CAD build for the part. Positions are in the model's coordinates, mm. Give positions to 0.01 mm unless a question says otherwise; leave off trailing zeros. Order: outer loops, then holes, each group sorted by start corner. A loop starts at its lowest first (then second) coordinate and runs counter-clockwise, first axis right, second up.
Item 1: Wall check: L1, parallel to Y at x = 14.5, z = 0.75; L2, parallel to Y at x = 23.5, z = 2.25; L3, parallel to X at y = 1.5, z = 6.5. Give the ranges that are in metal, low to high.
Item 2: Band-saw the part on A-A on z = 5.5. Give the cut face in (x, y) (3 decimals).
Item 3: Band-saw the part on D-D on x = 14. Give the cut face in (y, z) (3 decimals).
Item 4: Band-saw the part on B-B on x = 27. Give the cut face in (y, z), plus the area to 3 significant figures.
Item 5: Two-plate mould, pull along Y, no slides. Class faces 1 (the flat face through (14, 10, 4)), 2 (the flat face through (19.82, 12.146, 3.55)), 3 (the flat face through (26.8, 1.5, 3.5)), 4 (the flat face through (29.2, 6, 4)): released by +Y, released by -Y, zero draft, split by the parting line, or undercut.
Item 6: Band-saw the part on C-C on y = 2.3. Give the cut face in (x, z) (3 decimals), plus the area to 3 significant figures.
Item 7: Flat gauge pins, fed straight in: P1, Ø1, axis at x = 16.5, z = 2.5, coming from the +Y side; P2, Ø1.5, axis at x = 9.5, z = 1, coming from the +Y side; P3, Ø3.5, axis at x = 15.5, z = 4.5, coming from the +Y side. Where does each tip first touch, or does it go through?
Autodesk Inventor part; units mm, degrees
ref_plane "YZ Plane" through (0, 0, 0) normal (1, 0, 0) x (0, 1, 0)
ref_plane "XZ Plane" through (0, 0, 0) normal (0, 1, 0) x (-1, 0, 0)
ref_plane "XY Plane" through (0, 0, 0) normal (0, 0, 1) x (1, 0, 0)
sketch "スケッチ1" plane through (0, 0, 0) normal (0, 0, 1) x (1, 0, 0)
  line L0 (0, 0) -> (24.2856, 0)
  line L1 (29.2, 2.9323) -> (29.2, 10)
  line L2 (28.3778, 10) -> (0, 10)
  line L3 (0, 10) -> (0, 0)
  circle A0 centre (23.5, 2.3) radius 1.25
  circle A1 centre (14, 2.3) radius 1.175
  line L4 (29.2, 2.9323) -> (24.2856, 0)
  line L5 (29.2, 10) -> (11.5467, 14.4273)
  line L6 (11.5467, 14.4273) -> (11.4981, 14.2333)
  line L7 (11.4981, 14.2333) -> (28.3778, 10)
  dimension "d2" = 2.5
  dimension "d3" = 2.35
  dimension "d4" = 18.2
  dimension "d5" = 0.2
extrude "押し出し1" add sketch "スケッチ1" along normal blind 7.2
properties part number "microswitch" material "ABS プラスチック"
The answers:
1. L1: y = 0 to 1.24, 3.36 to 10, 13.48 to 13.69
1. L2: y = 0 to 1.05, 3.55 to 10, 11.22 to 11.43
1. L3: x = 0 to 13.14, 14.86 to 22.54, 24.46 to 26.8
2. outline: (0, 0) - (24.286, 0) - (29.2, 2.932) - (29.2, 10) - (11.547, 14.427) - (11.498, 14.233) - (28.378, 10) - (0, 10) - close; hole circle Ø2.35 at (14, 2.3); hole circle Ø2.5 at (23.5, 2.3)
3. outline: (0, 0) - (1.125, 0) - (1.125, 7.2) - (0, 7.2) - close; (3.475, 0) - (10, 0) - (10, 7.2) - (3.475, 7.2) - close; (13.606, 0) - (13.812, 0) - (13.812, 7.2) - (13.606, 7.2) - close
4. outline: (1.62, 0) - (10, 0) - (10, 7.2) - (1.62, 7.2) - close; (10.35, 0) - (10.55, 0) - (10.55, 7.2) - (10.35, 7.2) - close
4. area: 61.8 mm2
5. face 1: undercut
5. face 2: undercut
5. face 3: released by -Y
5. face 4: zero draft
6. outline: (0, 0) - (12.825, 0) - (12.825, 7.2) - (0, 7.2) - close; (15.175, 0) - (22.25, 0) - (22.25, 7.2) - (15.175, 7.2) - close; (24.75, 0) - (28.14, 0) - (28.14, 7.2) - (24.75, 7.2) - close
6. area: 168 mm2
7. P1: stops at y = 13.31
7. P2: stops at y = 10
7. P3: stops at y = 13.87
